Input: part model. Units: mm. Frame: model coordinates. A direction names the side the tool comes from. Round coordinates to 2 decimals unless told otherwise and drop trailing zeros. Write each loop counter-clockwise with the first axis right and the second up, starting at its lowest first coordinate (ties: lowest second). Pieces come first, ordered by that corner, then holes. Notation, with made-up numbers: (81, 73.25) -> (120, 73.25) arc R18 cw to (120, 83.25) -> close; hole circle Ø6 at (66, 82). An arc over 180 degrees is marked (long way). Use CSV: the item, a comma, the result in double quotes.
```python
from build123d import *

# Parameters (mm, degrees)
BOSS_EXTRUDE1_DEPTH              = 20
CUT_EXTRUDE1_START               = -4
SKETCH2_R                        = 1.625
CUT_EXTRUDE1_DEPTH               = 25
BOSS_EXTRUDE2_DEPTH              = 36.8
SKETCH8_R                        = 3
CUT_EXTRUDE5_DEPTH               = 19
CUT_EXTRUDE6_DEPTH               = 45
CUT_EXTRUDE7_REACH               = 42.8
CUT_EXTRUDE7_OFFSET_FROM_SURFACE = 4


with BuildPart() as part:
    # Sketch1 → Boss-Extrude1 (new body)
    with BuildSketch(Plane(origin=(0, 0, 0), x_dir=(1, 0, 0), z_dir=(0, 1, 0))):
        Polygon((0, 0), (18.4, 0), (18.4, 20), (31.8, 20), (31.8, 23), (13.4, 23), (13.4, 3), (0, 3), align=None)
    extrude(amount=BOSS_EXTRUDE1_DEPTH)

    # Sketch2 → Cut-Extrude1 (cut)
    with BuildSketch(Plane.XY.offset(-20).offset(CUT_EXTRUDE1_START)):
        with Locations((25.1, 17.5)):
            Circle(SKETCH2_R)
        with Locations((25.1, 2.8)):
            Circle(SKETCH2_R)
    cut_extrude1 = extrude(amount=CUT_EXTRUDE1_DEPTH, mode=Mode.SUBTRACT)

    # Mirror1: Cut-Extrude1 across plane
    add(cut_extrude1.mirror(Plane.ZY.offset(-15.9)), mode=Mode.SUBTRACT)

    # Sketch5 → Boss-Extrude2 (add)
    with BuildSketch(Plane.ZY):
        Polygon((0, 20), (0, -24), (18, -24), (14, 8), (14, 20), align=None)
        with BuildLine():
            Line((10.55, -9), (10.55, -19))
            ThreePointArc((10.55, -19), (8, -21.55), (5.45, -19))
            Line((5.45, -19), (5.45, -9))
            ThreePointArc((5.45, -9), (8, -6.45), (10.55, -9))
        make_face(mode=Mode.SUBTRACT)
    extrude(amount=-BOSS_EXTRUDE2_DEPTH)

    # Sketch8 → Cut-Extrude5 (cut, through all)
    with BuildSketch(Plane(origin=(0, 0, 0), x_dir=(-1, 0, 0), z_dir=(0, 0, -1))):
        with Locations((-6.7, 2.8)):
            Circle(SKETCH8_R)
        with Locations((-6.7, 17.5)):
            Circle(SKETCH8_R)
    extrude(amount=-CUT_EXTRUDE5_DEPTH, mode=Mode.SUBTRACT)

    # Sketch6 → Cut-Extrude6 (cut, through all)
    with BuildSketch(Plane.XZ.offset(24)):
        Polygon((36.8, 18), (36.8, 0), (36.730884622, 0), align=None)
    extrude(amount=-CUT_EXTRUDE6_DEPTH, mode=Mode.SUBTRACT)

    # Cut-Extrude7: up to this face of the body (flat: up to its plane, moved by the offset)
    cut_extrude7_end = Plane(part.part.faces().sort_by_distance((36.760677184, -1.783418912, 7.75899858))[0]).offset(-CUT_EXTRUDE7_OFFSET_FROM_SURFACE)
    # Sketch7 → Cut-Extrude7 (cut, up to the picked face)
    with BuildSketch(Plane.ZY, mode=Mode.PRIVATE) as cut_extrude7_sk1:
        with BuildLine():
            Line((14, -24), (14, -9))
            ThreePointArc((14, -9), (8, -3), (2, -9))
            Line((2, -9), (2, -24))
            Line((2, -24), (14, -24))
        make_face()
    cut_extrude7_tool1 = split(extrude(cut_extrude7_sk1.sketch, amount=-CUT_EXTRUDE7_REACH, mode=Mode.PRIVATE), bisect_by=cut_extrude7_end, keep=Keep.BOTH, mode=Mode.PRIVATE)
    add(cut_extrude7_tool1.solids().sort_by_distance((0, -14.098317, 8))[0], mode=Mode.SUBTRACT)


solid = part.part
```
Item 1: Pull-direction query (Z, two-part tool) for faces 1 (the face through (22, -7, 0)), 2 (the face through (0, 3, 7)), 3 (the face through (18, -8, 16)); classes: +Z half, -Z half, draft (parallel to the pull), parting line (faces both ways), or undercut.
Worked answers:
face 1,"undercut"
face 2,"draft"
face 3,"+Z half"
Item 2: Section query A-A on x = 25.1. Return the cut outline in (y, z) (3 decimals).
Worked answers:
outline,"(-24, 0) -> (20, 0) -> (20, 14) -> (8, 14) -> (-24, 18) -> (-24, 14) -> (-9, 14) arc R6 cw to (-9, 2) -> (-24, 2) -> close; (0, -23) -> (1.175, -23) -> (1.175, -20) -> (0, -20) -> close; (4.425, -23) -> (15.875, -23) -> (15.875, -20) -> (4.425, -20) -> close; (19.125, -23) -> (20, -23) -> (20, -20) -> (19.125, -20) -> close"
Item 3: Section query B-B on z = 8. Return the cut outline in (x, y), plus the area to 3 significant figures.
Worked answers:
outline,"(0, -3) -> (32.76, -3) -> (32.76, -6.45) -> (36.76, -6.45) -> (36.76, 20) -> (8.36, 20) arc R3 cw (long way) to (5.04, 20) -> (0, 20) -> close; (32.76, -24) -> (36.76, -24) -> (36.76, -21.55) -> (32.76, -21.55) -> close; hole circle Ø6 at (6.7, 2.8)"
area,"814 mm²"
Item 4: Set-up query: faces 4 (the face through (35, -14, 10.55)), 5 (the face through (31.8, 10, -21)), 6 (the face through (7, 10, -3)), 7 (the face through (5, 19, 0)). Return all of +Z, -Z, +X, -X, +Y, -Y with unobstructed straight access to the full face (end or side cutting, diameter ignored); none if empty.
Worked answers:
face 4,"+X, -X"
face 5,"-Z, +X, +Y, -Y"
face 6,"-Z, -X, +Y, -Y"
face 7,"+Z"
Item 5: Line query: line 1 (Y direction, x = 6.7, z = -1.2) (3 decimals); line 2 (X direction, y = 17.5, z = -21.4) (3 decimals); line 3 (Y direction, x = 6, z = -1). Output: solid intervals per line, ascending.
Worked answers:
line 1,"y = 0 to 1.175, 4.425 to 15.875, 19.125 to 20"
line 2,"x = 13.4 to 23.475, 26.725 to 31.8"
line 3,"y = 0 to 1.33, 4.27 to 16.03, 18.97 to 20"
Item 6: Section query D-D on x = 16. Return the cut outline in (y, z), plus the area to 3 significant figures.
Worked answers:
outline,"(-24, 0) -> (0, 0) -> (0, -23) -> (20, -23) -> (20, 14) -> (8, 14) -> (-24, 18) -> (-24, 14) -> (-9, 14) arc R6 cw to (-9, 2) -> (-24, 2) -> close"
area,"903 mm²"
Item 7: First-contact query: pin 1 Ø10 at (x, y) = (32, 10.5) entering from +Z; pin 2 Ø7 at (x, z) = (10.5, -9.5) entering from -Y; pin 3 Ø4 at (y, z) = (7.5, -12) entering from +X. Flat tips, straight axial feed; report the tip coordinate or a pass-through.
Worked answers:
pin 1,"stops at z = 14.31"
pin 2,"stops at y = 0"
pin 3,"stops at x = 18.4"
Item 8: Section query C-C on y = 17.5. Return the cut outline in (x, z) (3 decimals), plus the area to 3 significant figures.
Worked answers:
outline,"(0, -3) -> (5.075, -3) -> (5.075, 0) -> (3.7, 0) -> (3.7, 14) -> (0, 14) -> close; (8.325, -3) -> (13.4, -3) -> (13.4, -23) -> (23.475, -23) -> (23.475, -20) -> (18.4, -20) -> (18.4, 0) -> (36.731, 0) -> (36.785, 14) -> (9.7, 14) -> (9.7, 0) -> (8.325, 0) -> close; (26.725, -23) -> (31.8, -23) -> (31.8, -20) -> (26.725, -20) -> close"
area,"607 mm²"
